Input: part model. Units: mm. Frame: model coordinates. Face numbers are marked on the shaded views. A direction names the side the tool comes from. Round coordinates to 2 decimals unless told otherwise and drop trailing zeros. Write each loop counter-clockwise with the first axis right and the second up, starting at its lowest first coordinate (ties: lowest second). Pieces come first, ordered by that corner, then holes. Notation, with made-up numbers: M -23.5,-0.5 L 32.5,-0.5 A13 ccw 32.5,18.5 Z; hole C 19.5,14.25 d11. An arc over 180 degrees is marked long. Write each question's results on one line, items separated by ' | '. Start each with the question number.
```python
from build123d import *

# Parameters (mm, degrees)
F0_W     = 76.2
F0_H     = 152.4
F1_DEPTH = 50.8
F3_D     = 5.1054
F5_D     = 5.1054
F6_W     = 71.12
F6_H     = 45.72
F7_DEPTH = 152.4


with BuildPart() as f1:
    # F0 (on Top) → F1 (new body)
    with BuildSketch(Plane.XY):
        with Locations((3.184349, -12.893389)):
            Rectangle(F0_W, F0_H)
    extrude(amount=F1_DEPTH)

    # F3 (through all)
    with Locations(Plane.XY.offset(50.8)):
        with Locations((-22.215651, -0.193389), (28.584349, -0.193389), (3.184349, -50.993389), (3.184349, -25.593389), (28.584349, -50.993389), (28.584349, -25.593389), (28.584349, 25.206611), (28.584349, -76.393389), (3.184349, 50.606611), (3.184349, -76.393389), (28.584349, 50.606611), (3.184349, -0.193389), (3.184349, 25.206611), (-22.215651, 25.206611), (-22.215651, -76.393389), (-22.215651, 50.606611), (-22.215651, -25.593389), (-22.215651, -50.993389)):
            Hole(F3_D / 2)

    # F5 (through all)
    with Locations(Plane.YZ.offset(41.284349)):
        with Locations((-25.593389, 38.1), (-0.193389, 12.7), (-50.993389, 38.1), (-25.593389, 12.7), (50.606611, 12.7), (50.606611, 38.1), (-0.193389, 38.1), (25.206611, 12.7), (-50.993389, 12.7), (-76.393389, 12.7), (-76.393389, 38.1), (25.206611, 38.1)):
            Hole(F5_D / 2)

    # F6 (on face) → F7 (cut)
    with BuildSketch(Plane(origin=(0, 63.306611, 0), x_dir=(-1, 0, 0), z_dir=(0, 1, 0))):
        with Locations((-3.184349, 25.4)):
            Rectangle(F6_W, F6_H)
    extrude(amount=-F7_DEPTH, mode=Mode.SUBTRACT)


solid = f1.part
```
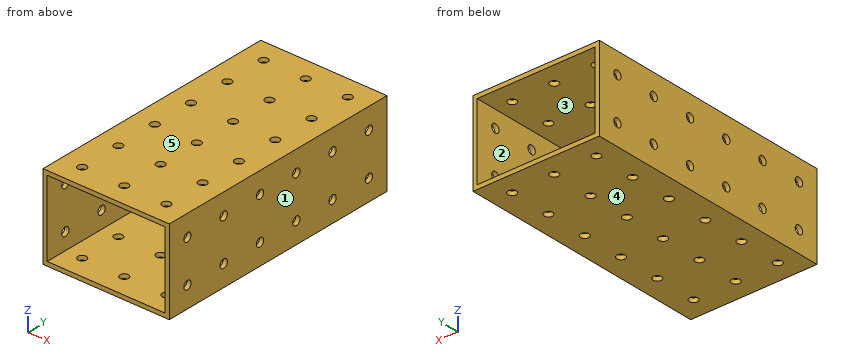
1. Contact query for a flat-ended pin moving along its axis: P1, Ø6.5, axis at x = 3.18, y = -25.59, coming from the -Z side. Output: stop coordinate, or through.
2. Draft query along Z for the marked faces 3, 4 and 5. Return one class per face: +Z half, -Z half, draft (parallel to the pull), parting line (faces both ways), or undercut.
3. Cut plane A-A on y = -4.5. Output: boundary loops of the cut face in (x, z), and give its area (3 significant figures).
4. Cut plane D-D on z = 12.7. Give the number of separate pieces and of enclosed holes in the cut face, and give its area (3 significant figures).
5. Cut plane C-C on z = 32. Output: boundary loops of the cut face in (x, y), and give its area (3 significant figures).
6. Access query for the marked faces 1 and 2. Directions: +Z, -Z, +X, -X, +Y, -Y. A direction counts if a zero-diameter tool reaches every point of the face in a straight line with its end or side. Return the directions, or none.
7. Cut plane B-B on x = 16.5. Output: boundary loops of the cut face in (y, z), and give its area (3 significant figures).
8. Line query: L1, parallel to Z at x = -15.5, y = -71.5; L2, parallel to X at y = -34, z = 25.5. Output: solid intervals per line, ascending. Write a range as from..to.
Answers follow:
1) P1: stops at z = 0
2) face 3: undercut | face 4: -Z half | face 5: +Z half
3) outline: M -34.92,0 L 41.28,0 L 41.28,50.8 L -34.92,50.8 Z; hole M -32.38,2.54 L 38.74,2.54 L 38.74,48.26 L -32.38,48.26 Z | area: 619 mm2
4) separate pieces: 14 | enclosed holes: 0 | area: 619 mm2
5) outline: M -34.92,-89.09 L -32.38,-89.09 L -32.38,63.31 L -34.92,63.31 Z; M 38.74,-89.09 L 41.28,-89.09 L 41.28,63.31 L 38.74,63.31 Z | area: 774 mm2
6) face 1: +Z, -Z, +X, +Y, -Y | face 2: +Y, -Y
7) outline: M -89.09,0 L 63.31,0 L 63.31,2.54 L -89.09,2.54 Z; M -89.09,48.26 L 63.31,48.26 L 63.31,50.8 L -89.09,50.8 Z | area: 774 mm2
8) L1: z = 0..2.54, 48.26..50.8 | L2: x = -34.92..-32.38, 38.74..41.28
